For this review, take the finished solid that the model builds, in its own axes (mm). A direction names the side the tool comes from. Coordinates: 2 decimals unless noted, no trailing zeros. Write each loop counter-clockwise with the first axis right and the second up, starting at its lowest first coordinate (ties: lowest second). Pieces come first, ordered by that corner, then holes.
```python
from build123d import *

# Parameters (mm, degrees)
SKETCH_1_R          = 1.5
SKETCH_1_W          = 24
SKETCH_1_H          = 15
EXTRUDE_1_DEPTH     = 3
SKETCH_2_R          = 2
SKETCH_2_R_2        = 1.5
EXTRUDE_2_DEPTH     = 1
CUT_EXTRUDE_1_REACH = 41.246
SKETCH_3_W          = 7
SKETCH_3_H          = 3
FILLET_1_R          = 8


with BuildPart() as part:
    # 草图1 → 凸台-拉伸1 (new body)
    with BuildSketch(Plane(origin=(0, 0, 0), x_dir=(1, 0, 0), z_dir=(0, 1, 0))):
        Polygon((-14, -8.5), (0, -8.5), (0, -17.5), (35, -17.5), (35, 17.5), (0, 17.5), (0, 8.5), (-14, 8.5), (-21, 8.5), (-21, -8.5), align=None)
        with Locations(Location((-2.5, 0, 0), (0, 0, 270))):
            Circle(SKETCH_1_R, mode=Mode.SUBTRACT)
        with Locations(Location((29.5, -12.5, 0), (0, 0, 270))):
            Circle(SKETCH_1_R, mode=Mode.SUBTRACT)
        with Locations(Location((5.5, -12.5, 0), (0, 0, 270))):
            Circle(SKETCH_1_R, mode=Mode.SUBTRACT)
        with Locations(Location((29.5, 12.5, 0), (0, 0, 270))):
            Circle(SKETCH_1_R, mode=Mode.SUBTRACT)
        with Locations(Location((5.5, 12.5, 0), (0, 0, 270))):
            Circle(SKETCH_1_R, mode=Mode.SUBTRACT)
        with Locations(Location((-17.5, -5, 0), (0, 0, 270))):
            Circle(SKETCH_1_R, mode=Mode.SUBTRACT)
        with Locations(Location((-17.5, 5, 0), (0, 0, 270))):
            Circle(SKETCH_1_R, mode=Mode.SUBTRACT)
        with Locations((17.5, 0)):
            Rectangle(SKETCH_1_W, SKETCH_1_H, mode=Mode.SUBTRACT)
    extrude(amount=EXTRUDE_1_DEPTH)

    # 草图2 → 凸台-拉伸2 (add)
    # profile 1 of 4: a face of its own
    with BuildSketch(Plane(origin=(0, 3, 0), x_dir=(1, 0, 0), z_dir=(0, 1, 0))):
        with Locations(Location((5.5, 12.5, 0), (0, 0, 270))):
            Circle(SKETCH_2_R)
        with Locations(Location((5.5, 12.5, 0), (0, 0, 270))):
            Circle(SKETCH_2_R_2, mode=Mode.SUBTRACT)
    # profile 2 of 4: a face of its own
    with BuildSketch(Plane(origin=(0, 3, 0), x_dir=(1, 0, 0), z_dir=(0, 1, 0))):
        with Locations(Location((29.5, 12.5, 0), (0, 0, 270))):
            Circle(SKETCH_2_R)
        with Locations(Location((29.5, 12.5, 0), (0, 0, 270))):
            Circle(SKETCH_2_R_2, mode=Mode.SUBTRACT)
    # profile 3 of 4: a face of its own
    with BuildSketch(Plane(origin=(0, 3, 0), x_dir=(1, 0, 0), z_dir=(0, 1, 0))):
        with Locations(Location((29.5, -12.5, 0), (0, 0, 270))):
            Circle(SKETCH_2_R)
        with Locations(Location((29.5, -12.5, 0), (0, 0, 270))):
            Circle(SKETCH_2_R_2, mode=Mode.SUBTRACT)
    # profile 4 of 4: a face of its own
    with BuildSketch(Plane(origin=(0, 3, 0), x_dir=(1, 0, 0), z_dir=(0, 1, 0))):
        with Locations(Location((5.5, -12.5, 0), (0, 0, 270))):
            Circle(SKETCH_2_R)
        with Locations(Location((5.5, -12.5, 0), (0, 0, 270))):
            Circle(SKETCH_2_R_2, mode=Mode.SUBTRACT)
    extrude(amount=EXTRUDE_2_DEPTH)

    # 草图3 → 切除-拉伸1 (cut, up to next)
    with BuildSketch(Plane(origin=(0, 3, 0), x_dir=(1, 0, 0), z_dir=(0, 1, 0)), mode=Mode.PRIVATE) as cut_extrude_1_sk1:
        with Locations((-17.5, 0)):
            Rectangle(SKETCH_3_W, SKETCH_3_H)
    cut_extrude_1_tool1 = extrude(cut_extrude_1_sk1.sketch, amount=-CUT_EXTRUDE_1_REACH, mode=Mode.PRIVATE) & part.part
    add(cut_extrude_1_tool1.solids().sort_by_distance((-17.5, 3, 0))[0], mode=Mode.SUBTRACT)

    # 圆角1
    fillet_1_edges = [part.edges().sort_by_distance(p)[0] for p in [
        (0, 1.5, -17.5),
        (35, 1.5, -17.5),
        (35, 1.5, 17.5),
        (0, 1.5, 17.5),
    ]]
    fillet(fillet_1_edges, radius=FILLET_1_R)


solid = part.part
```
Q1. Add section A-A (z = 0). State the section outline as (x, y) points, then the cut area to 3 significant figures.
Ans:
outline: (-14, 0) - (-4, 0) - (-4, 3) - (-14, 3) - close; (-1, 0) - (5.5, 0) - (5.5, 3) - (-1, 3) - close; (29.5, 0) - (35, 0) - (35, 3) - (29.5, 3) - close
area: 66.0 mm2
Q2. Add section B-B (x = 12). State the section outline as (y, z) points.
Ans:
outline: (0, -17.5) - (3, -17.5) - (3, -7.5) - (0, -7.5) - close; (0, 7.5) - (3, 7.5) - (3, 17.5) - (0, 17.5) - close
Q3. Add section D-D (z = -5). State the section outline as (x, y) points.
Ans:
outline: (-21, 0) - (-19, 0) - (-19, 3) - (-21, 3) - close; (-16, 0) - (5.5, 0) - (5.5, 3) - (-16, 3) - close; (29.5, 0) - (35, 0) - (35, 3) - (29.5, 3) - close
Q4. For probe 1 along X at (y, z) = (2.1, 5); probe 2 along Z at (x, y) = (5, 0.35); probe 3 along X at (y, z) = (3.1, -12.5), list the stretches that pass through material, from the lowest coordinate up.
Ans:
probe 1: x = -21 to -19, -16 to 5.5, 29.5 to 35
probe 2: z = -16.92 to -13.91, -11.09 to 11.09, 13.91 to 16.92
probe 3: x = 3.5 to 4, 7 to 7.5, 27.5 to 28, 31 to 31.5
Q5. Tool access review of faces 4 (the cylindrical face through (2.406, 1.521, 15.219)), 5 (the flat face through (5.5, 1, 0)), 6 (the flat face through (-14, 2, 0)), 7 (the flat face through (-10, 1, -8.5)): name each direction out of +Z, -Z, +X, -X, +Y, -Y from which nothing blocks a thin tool from reaching the whole face with its end or side.
Ans:
face 4: +Z, -X, +Y, -Y
face 5: +Y, -Y
face 6: -X, +Y, -Y
face 7: -Z, -X, +Y, -Y
Q6. Add section C-C (y = 2.45). Give the number of separate pieces and of enclosed holes in the cut face, then the cut area to 3 significant figures.
Ans:
separate pieces: 1
enclosed holes: 8
area: 1,100 mm2
Q7. Clearance check with flat-ended pins moving along their axes: pin 1 Ø2.5 at (x, z) = (29.5, -12.5) entering from -Y; pin 2 Ø2 at (x, z) = (0.5, -13) entering from +Y; pin 3 Ø0.9 at (x, y) = (-9, 2) entering from +Z; pin 4 Ø1.5 at (y, z) = (3, 11.5) entering from -X. State where each tip first meets the part, or that it passes through.
Ans:
pin 1: passes through
pin 2: stops at y = 3
pin 3: stops at z = 8.5
pin 4: stops at x = 0.1
Q8. Draft analysis for pull direction Z (two halves, no side actions). For faces 1 (the cylindrical face through (6.852, 3.493, -13.974)), 2 (the flat face through (-11, 1, 8.5)), 3 (the flat face through (13, 0, 8)), state which applies: +Z half, -Z half, draft (parallel to the pull), parting line (faces both ways), or undercut.
Ans:
face 1: undercut
face 2: +Z half
face 3: draft
